from build123d import *

# Parameters (mm, degrees)
BOSS_EXTRUDE1_DEPTH = 0.7
NOTCH_DEPTH         = 0.7


with BuildPart() as part:
    # Sketch3 → Boss-Extrude1 (new body)
    with BuildSketch(Plane(origin=(0, 0, 0), x_dir=(1, 0, 0), z_dir=(0, 1, 0))):
        with BuildLine():
            Line((-70.309797243, 11.349925621), (-83.143655207, 13.421661553))
            ThreePointArc((-83.143655207, 13.421661553), (-6.732375453, -83.950482552), (84.22, 0))
            Line((84.22, 0), (71.22, 0))
            ThreePointArc((71.22, 0), (-5.693181902, -70.992084628), (-70.309797243, 11.349925621))
        make_face()
    extrude(amount=BOSS_EXTRUDE1_DEPTH)

    # Sketch4 → notch (add)
    with BuildSketch(Plane(origin=(0, 0, 0), x_dir=(1, 0, 0), z_dir=(0, 1, 0))):
        Polygon((83, 1.400205806), (72.5, 1.308573694), (72.5, 0), (83, 0), align=None)
        with BuildLine():
            Line((83.400376749, 11.721158563), (70.526891856, 9.91190825))
            ThreePointArc((70.526891856, 9.91190825), (70.998315276, 5.614946842), (71.208183604, 1.297300183))
            Line((71.208183604, 1.297300183), (72.5, 1.308573694))
            Line((72.5, 1.308573694), (83, 1.400205806))
            Line((83, 1.400205806), (84.208183604, 1.410749464))
            ThreePointArc((84.208183604, 1.410749464), (83.962691178, 6.578365305), (83.400376749, 11.721158563))
        make_face()
    notch = extrude(amount=NOTCH_DEPTH)

    # Mirror1: notch across plane
    add(notch.mirror(Plane(origin=(0, 0, 0), x_dir=(-0.07993796548331146, 0, 0.9967998403262256), z_dir=(-0.9967998403262257, 0, -0.07993796548331145))))


solid = part.part
Geometry check sheet. Reference: the model listing, model coordinates, mm. Give positions to 0.01 mm unless a question says otherwise; leave off trailing zeros. Loops run counter-clockwise (first coordinate to the right, second up) from the corner with the lowest first, then second, coordinate; pieces in that order, holes last. Notation, with made-up numbers: (-30, 37) -> (-13, 37) arc R21 ccw to (-13, 48) -> close; hole circle Ø5 at (71, 33). An arc over 180 degrees is marked (long way). Answer in a Markdown table with one row per item. Add a question column.
1) Gauge pin test, flat end, axial feed: P1, Ø12, axis at x = -66, z = 8, coming from the +Y side. Record the tip position at first contact, or that the pin passes through.
2) Cross-section at C-C on z = 15. Record the boundary of the cut face in (x, y).
3) Cross-section at B-B on z = 36.5. Record the boundary of the cut face in (x, y).
4) Cross-section at D-D on x = 0. Record the boundary of the cut face in (y, z), and give its area (3 significant figures).
5) Cross-section at A-A on y = 0.15. Record the boundary of the cut face in (x, z), and give its area (3 significant figures).
6) Material ranges on probe 1 along X at (y, z) = (0.45, 58); probe 2 along Z at (x, y) = (0, 0.2); probe 3 along X at (y, z) = (0.5, 55), recorded low to high. Write a range as from..to.
Outcome:
| question | item | result |
|---|---|---|
| 1 | P1 | stops at y = 0.7 |
| 2 | outline | (-82.87, 0) -> (-69.62, 0) -> (-69.62, 0.7) -> (-82.87, 0.7) -> close; (69.62, 0) -> (82.87, 0) -> (82.87, 0.7) -> (69.62, 0.7) -> close |
| 3 | outline | (-75.9, 0) -> (-61.16, 0) -> (-61.16, 0.7) -> (-75.9, 0.7) -> close; (61.16, 0) -> (75.9, 0) -> (75.9, 0.7) -> (61.16, 0.7) -> close |
| 4 | outline | (0, 71.22) -> (0.7, 71.22) -> (0.7, 84.22) -> (0, 84.22) -> close |
| 4 | area | 9.10 mm^2 |
| 5 | outline | (-83.14, -13.42) -> (-81.94, -13.23) -> (-81.72, -14.61) -> (-82.91, -14.81) arc R84.22 ccw to (-80.47, -24.86) -> (-68.05, -21.02) arc R71.22 cw to (-70.09, -12.63) -> (-71.36, -12.85) -> (-71.57, -11.55) -> (-70.31, -11.35) arc R71.22 cw (long way) to (71.22, 0) -> (72.5, 0) -> (72.5, -1.31) -> (71.21, -1.3) arc R71.22 cw to (70.53, -9.91) -> (83.4, -11.72) arc R84.22 ccw to (84.21, -1.41) -> (83, -1.4) -> (83, 0) -> (84.22, 0) arc R84.22 ccw (long way) to start |
| 5 | area | 3,610 mm^2 |
| 6 | probe 1 | x = -61.07..-41.33, 41.33..61.07 |
| 6 | probe 2 | z = 71.22..84.22 |
| 6 | probe 3 | x = -63.78..-45.25, 45.25..63.78 |
